from build123d import *

# Parameters (mm, degrees)
SKETCH1_R                = 16
SKETCH1_R_2              = 11.4
BOSS_EXTRUDE1_DEPTH      = 20
SKETCH2_R                = 16
BOSS_EXTRUDE2_DEPTH      = 2
BOSS_EXTRUDE3_DEPTH      = 16
BOSS_EXTRUDE3_DEPTH_BACK = 16
CUT_EXTRUDE1_DEPTH       = 30.002175046
BOSS_EXTRUDE4_REACH      = 31.002
SKETCH5_R                = 16
SKETCH6_R                = 4.05
CUT_EXTRUDE3_DEPTH       = 29.757190977


with BuildPart() as part:
    # Sketch1 → Boss-Extrude1 (new body)
    with BuildSketch(Plane.XY):
        Circle(SKETCH1_R)
        Circle(SKETCH1_R_2, mode=Mode.SUBTRACT)
    extrude(amount=BOSS_EXTRUDE1_DEPTH)

    # Sketch2 → Boss-Extrude2 (add)
    with BuildSketch(Plane(origin=(0, 0, 0), x_dir=(-1, 0, 0), z_dir=(0, 0, -1))):
        Circle(SKETCH2_R)
    extrude(amount=BOSS_EXTRUDE2_DEPTH)

    # Sketch3 → Boss-Extrude3 (add, two sides)
    with BuildSketch(Plane(origin=(0, 0, 0), x_dir=(0, 0, -1), z_dir=(1, 0, 0))) as boss_extrude3_sk:
        Polygon((31.002175046, 25.419398483), (26.906414824, 28.287280664), (18.302768279, 16), (2, -7.282766022), (2, -16), align=None)
    extrude(amount=BOSS_EXTRUDE3_DEPTH)
    extrude(boss_extrude3_sk.sketch, amount=-BOSS_EXTRUDE3_DEPTH_BACK)

    # Sketch4 → Cut-Extrude1 (cut, through all)
    with BuildSketch(Plane(origin=(0, 0, -2), x_dir=(-1, 0, 0), z_dir=(0, 0, -1))):
        with BuildLine():
            Line((34.266518051, 0), (16, 0))
            ThreePointArc((16, 0), (15.555436181, -3.745451268), (14.24644935, -7.282766022))
            ThreePointArc((14.24644935, -7.282766022), (0, -16), (-14.24644935, -7.282766022))
            ThreePointArc((-14.24644935, -7.282766022), (-15.555436181, -3.745451268), (-16, 0))
            Line((-16, 0), (-34.430612934, 0))
            Line((-34.430612934, 0), (-36.46308972, -20.488677285))
            Line((-36.46308972, -20.488677285), (32.179774964, -27.298049462))
            Line((32.179774964, -27.298049462), (34.266518051, 0))
        make_face()
    extrude(amount=CUT_EXTRUDE1_DEPTH, mode=Mode.SUBTRACT)

    # Sketch5 → Boss-Extrude4 (add, up to next)
    with BuildSketch(Plane(origin=(0, 0, -2), x_dir=(-1, 0, 0), z_dir=(0, 0, -1)), mode=Mode.PRIVATE) as boss_extrude4_sk1:
        Circle(SKETCH5_R)
    boss_extrude4_tool1 = extrude(boss_extrude4_sk1.sketch, amount=BOSS_EXTRUDE4_REACH, mode=Mode.PRIVATE) - part.part
    add(boss_extrude4_tool1.solids().sort_by_distance((0, 0, -2))[0])

    # Sketch6 → Cut-Extrude3 (cut, through all)
    with BuildSketch(Plane(origin=(0, -3.335649292, -4.763800888), x_dir=(1, 0, 0), z_dir=(0, 0.573576436, 0.819152044))):
        with Locations((0, 31.104469313)):
            Circle(SKETCH6_R)
    extrude(amount=-CUT_EXTRUDE3_DEPTH, mode=Mode.SUBTRACT)


solid = part.part
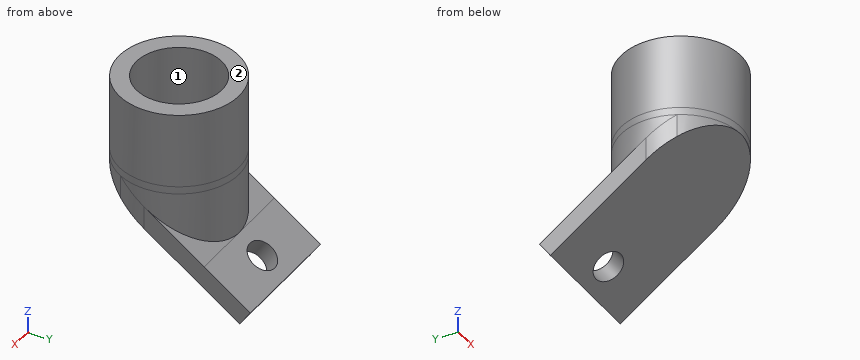
Build history of the part. All positions in model axes, mm. Face numbers are marked on the shaded views. Round coordinates to 2 decimals unless told otherwise and drop trailing zeros. Loops run counter-clockwise (first coordinate to the right, second up) from the corner with the lowest first, then second, coordinate; pieces in that order, holes last. Notation, with made-up numbers: (79, 77.25) -> (129, 77.25) arc R9 ccw to (129, 90.25) -> close; hole circle Ø11 at (4.5, 63). An arc over 180 degrees is marked (long way). One line per item, written item: value. Start each with the question number.
Q1. Cut at B-B on z = 3. List the corners of the cut face in (x, y).
Q2. Drop flat-ended pins along their axis: pin 1 Ø6 at (x, y) = (1.5, 21) entering from -Z; pin 2 Ø4 at (y, z) = (8, -22.5) entering from +X; pin 3 Ø2 at (y, z) = (3.5, -8.5) entering from +X; pin 4 Ø1 at (y, z) = (-5, -9) entering from +X. Give the stop position or say it passes through.
Q3. Cut at C-C on y = 12. List the corners of the cut face in (x, z).
Q4. Cut at A-A on x = -9.5. List the corners of the cut face in (y, z), plus the area to 3 significant figures.
Q5. Probe line 1 along Y through (x, z) = (0, 5); line 2 along X through (y, z) = (1, 17.5); line 3 along X through (y, z) = (-8, 11.5). List the from-to ranges inside material, lowest first.
Q6. Two-plate mould, pull along X, no slides. Class the marked faces 1 and 2: released by +X, released by -X, zero draft, split by the parting line, or undercut.
Q7. Cut at D-D on z = -10. List the corners of the cut face in (x, y).
Computed:
1. outline: circle Ø32 at (0, 0); hole circle Ø22.8 at (0, 0)
2. pin 1: z = -30.01
2. pin 2: through
2. pin 3: x = 16
2. pin 4: x = 15.35
3. outline: (-16, -21.61) -> (16, -21.61) -> (16, -15.5) -> (10.58, -15.5) -> (10.58, 20) -> (-10.58, 20) -> (-10.58, -15.5) -> (-16, -15.5) -> close
4. outline: (-12.87, -4.19) -> (25.42, -31) -> (28.29, -26.91) -> (12.87, -16.11) -> (12.87, 20) -> (6.3, 20) -> (6.3, 0) -> (-6.3, 0) -> (-6.3, 20) -> (-12.87, 20) -> close
4. area: 688 mm²
5. line 1: -16 to -11.4, 11.4 to 16
5. line 2: -15.97 to -11.36, 11.36 to 15.97
5. line 3: -13.86 to -8.12, 8.12 to 13.86
6. face 1: undercut
6. face 2: zero draft
7. outline: (-16, 0) arc R16 ccw to (-15.33, -4.57) -> (15.33, -4.57) arc R16 ccw to (16, 0) -> (16, 4.14) -> (15.45, 4.14) arc R16 ccw to (-15.45, 4.14) -> (-16, 4.14) -> close
